Design review of the part shown in the three views and the two pictorial views. Dimensions are in mm from the part's minimum x, y and z. A direction names the side the tool comes from. Round coordinates to 2 decimals unless told otherwise and drop trailing zeros. Loops run counter-clockwise (first coordinate to the right, second up) from the corner with the lowest first, then second, coordinate; pieces in that order, holes last. Notation, with made-up numbers: M 49.5,4.25 L 107.5,4.25 A23 ccw 107.5,21.25 Z; hole C 64.5,17.25 d3. An arc over 180 degrees is marked long. One line per question, with ' | ' between items.
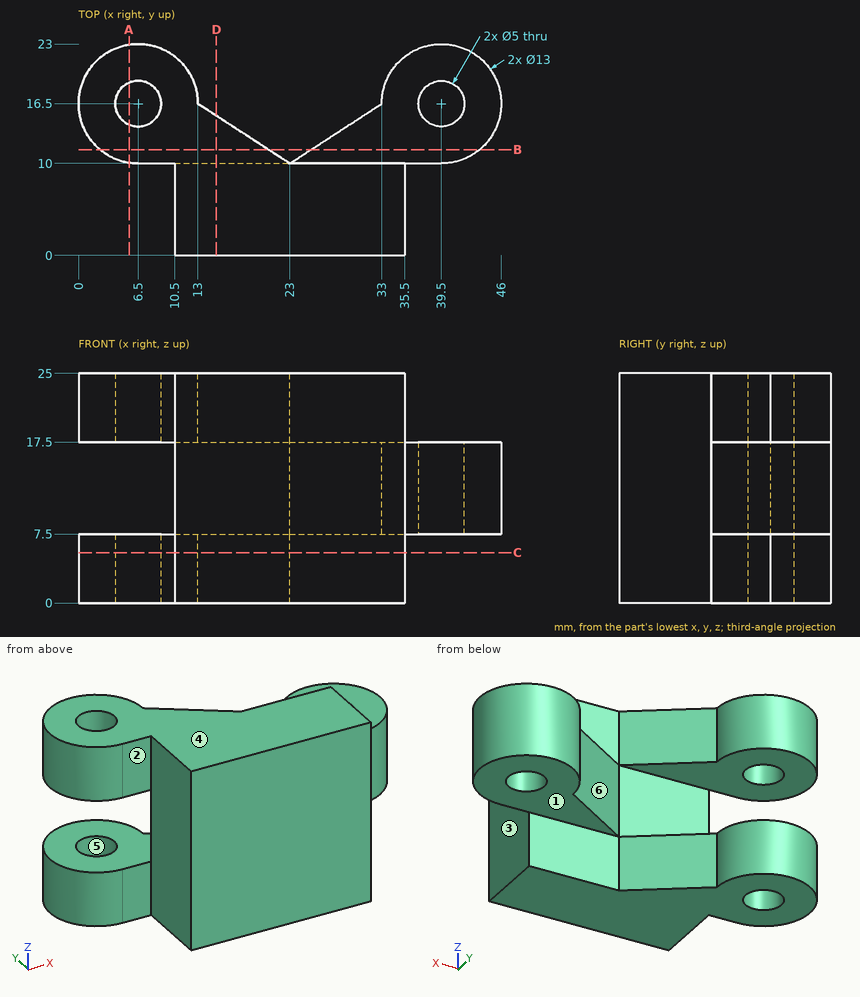
1) Mouldability with a two-part tool opening along X and no side actions: class the marked faces 4, 5 and 6 as +X half, -X half, draft (parallel to the pull), parting line (faces both ways), or undercut.
Output values:
face 4: draft | face 5: undercut | face 6: -X half
2) Machinability: for the marked faces 1, 2 and 3, which of the approach directions +Z, -Z, +X, -X, +Y, -Y give a long, thin tool a straight path to every point of the face, cutting with its end or side? Answer none if there is none.
Output values:
face 1: -Z, +X, +Y | face 2: +Z, -Z, -X, -Y | face 3: +Z, -Z, +X, -Y
3) For line 1 (Y direction, x = 6.5, z = 5); line 2 (Z direction, x = 9.5, y = 16.25); line 3 (X direction, y = 5, z = 6), list the stretches that pass through material, from the lowest coordinate up.
Output values:
line 1: y = 10 to 14, 19 to 23 | line 2: z = 0 to 7.5, 17.5 to 25 | line 3: x = 10.5 to 35.5
4) Add section B-B on y = 11.5. State the section outline as (x, z) points.
Output values:
outline: M 2.35,0 L 20.69,0 L 20.69,7.5 L 2.35,7.5 Z; M 2.35,17.5 L 20.69,17.5 L 20.69,25 L 2.35,25 Z; M 25.31,7.5 L 43.65,7.5 L 43.65,17.5 L 25.31,17.5 Z
5) Add section D-D on x = 15. State the section outline as (y, z) points, then the cut area to 3 significant figures.
Output values:
outline: M 0,0 L 15.2,0 L 15.2,7.5 L 10,7.5 L 10,17.5 L 15.2,17.5 L 15.2,25 L 0,25 Z | area: 328 mm²
6) Insertion check: P1, Ø3, axis at x = 18, z = 2.5, coming from the +Y side (3 decimals); P2, Ø8, axis at y = 5.5, z = 18, coming from the -X side; P3, Ø1, axis at y = 11.5, z = 17.5, coming from the +X side. Each pin has a flat end and moves straight along its axis. Give the tip position at first contact, or say it passes through.
Output values:
P1: stops at y = 14.225 | P2: stops at x = 10.5 | P3: stops at x = 44.19
7) Add section A-A on x = 5.5. State the section outline as (y, z) points, then the cut area to 3 significant figures.
Output values:
outline: M 10.08,0 L 14.21,0 L 14.21,7.5 L 10.08,7.5 Z; M 10.08,17.5 L 14.21,17.5 L 14.21,25 L 10.08,25 Z; M 18.79,0 L 22.92,0 L 22.92,7.5 L 18.79,7.5 Z; M 18.79,17.5 L 22.92,17.5 L 22.92,25 L 18.79,25 Z | area: 124 mm²
8) Add section C-C on z = 5.5. State the section outline as (x, y) points, then the cut area to 3 significant figures.
Output values:
outline: M 6.5,10 L 10.5,10 L 10.5,0 L 35.5,0 L 35.5,10 L 23,10 L 13,16.5 A6.5 ccw long Z; hole C 6.5,16.5 d5 | area: 405 mm²
